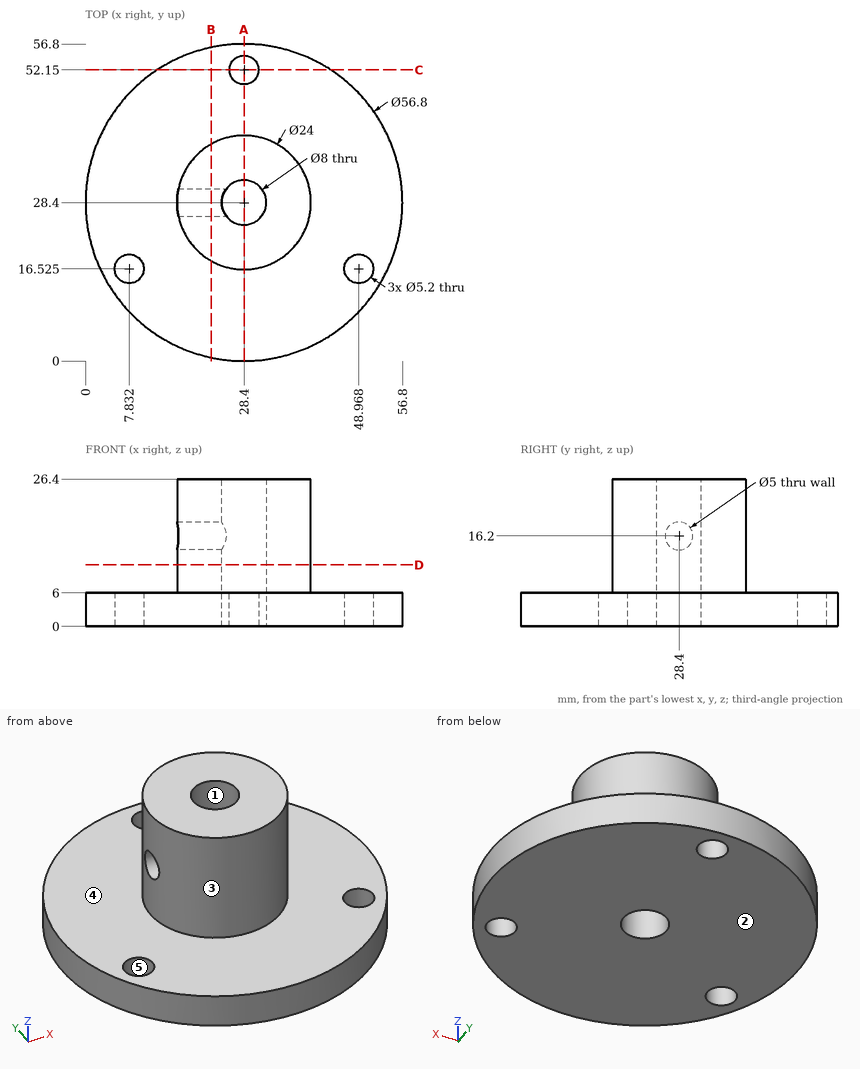
For this review, use the dimensioned drawing (mm, ordinates from the lowest corner) and the shaded views. A direction names the side the tool comes from. Give positions to 0.01 mm unless a question says otherwise; leave off trailing zeros. Order: outer loops, then holes, each group sorted by start corner. A loop starts at its lowest first (then second) coordinate and runs counter-clockwise, first axis right, second up. Notation, with made-up numbers: M 70,48.25 L 100,48.25 A17 ccw 100,64.25 Z; hole C 79,10 d11. An arc over 180 degrees is marked long. One line per question, with ' | ' between items. Start each with the question number.
1) Consider section C-C, the plane y = 52.15. Give the boundary of the cut face in (x, z), then the cut area to 3 significant figures.
2) Mouldability with a two-part tool opening along X and no side actions: class the marked faces 1, 2 and 3 as pulls with the +X half, pulls with the -X half, needs draft (parallel to the pull), parting line crosses it, or undercut.
3) For the marked faces 4 and 5, list the 3-axis set-ups (+Z, -Z, +X, -X, +Y, -Y) from which the entire face can be reached by the end or side of a thin tool; tool diameter is ignored.
4) Wall thickness on L1, parallel to Y at x = 28.4, z = 3.9; L2, parallel to Y at x = 28.4, z = 17.75; L3, parallel to Z at x = 49, y = 35.5: over which ranges is each line inside the solid? List them lowest first. Write a range as from..to.
5) Consider section A-A, the plane x = 28.4. Give the boundary of the cut face in (y, z), then the cut area to 3 significant figures.
6) Clearance check with flat-ended pins moving along their axes: P1, Ø6, axis at x = 12.5, z = 5.5, coming from the -Y side; P2, Ø10, axis at x = 43, z = 13.5, coming from the -Y side; P3, Ø6.5, axis at y = 28.4, z = 16.2, coming from the -X side. State where each tip first meets the part, or that it passes through.
7) Consider section B-B, the plane x = 22.5. Give the boundary of the cut face in (y, z), then the cut area to 3 significant figures.
8) Consider section D-D, the plane z = 11. Give the boundary of the cut face in (x, y).
Found:
1) outline: M 12.83,0 L 25.8,0 L 25.8,6 L 12.83,6 Z; M 31,0 L 43.97,0 L 43.97,6 L 31,6 Z | area: 156 mm²
2) face 1: undercut | face 2: needs draft | face 3: parting line crosses it
3) face 4: +Z | face 5: +Z, -Z
4) L1: y = 0..24.4, 32.4..49.55, 54.75..56.8 | L2: y = 16.4..24.4, 32.4..40.4 | L3: z = 0..6
5) outline: M 0,0 L 24.4,0 L 24.4,26.4 L 16.4,26.4 L 16.4,6 L 0,6 Z; M 32.4,0 L 49.55,0 L 49.55,6 L 40.4,6 L 40.4,26.4 L 32.4,26.4 Z; M 54.75,0 L 56.8,0 L 56.8,6 L 54.75,6 Z | area: 588 mm²
6) P1: stops at y = 3.1 | P2: stops at y = 21.2 | P3: stops at x = 16.4
7) outline: M 0.62,0 L 56.18,0 L 56.18,6 L 38.85,6 L 38.85,26.4 L 17.95,26.4 L 17.95,6 L 0.62,6 Z; hole C 28.4,16.2 d5 | area: 740 mm²
8) outline: C 28.4,28.4 d24; hole C 28.4,28.4 d8
